```python
from build123d import *

# Parameters (mm, degrees)
SKETCH1_R           = 18.5
BOSS_EXTRUDE1_DEPTH = 21.56
SKETCH2_R           = 6
BOSS_EXTRUDE2_DEPTH = 6
SKETCH3_R           = 3
BOSS_EXTRUDE3_DEPTH = 15
SKETCH4_R           = 1.5
CUT_EXTRUDE1_DEPTH  = 4
SKETCH5_R           = 16.4
BOSS_EXTRUDE4_DEPTH = 34
SKETCH7_R           = 0.75
BOSS_EXTRUDE5_DEPTH = 10
SKETCH8_R           = 0.75
BOSS_EXTRUDE6_DEPTH = 10


with BuildPart() as part:
    # Sketch1 → Boss-Extrude1 (new body)
    with BuildSketch(Plane.XY):
        with Locations((-38.660623091, 1.939719844)):
            Circle(SKETCH1_R)
    extrude(amount=BOSS_EXTRUDE1_DEPTH)

    # Sketch2 → Boss-Extrude2 (add)
    with BuildSketch(Plane.XY.offset(21.56)):
        with Locations((-41.618854638, 10.439653144)):
            Circle(SKETCH2_R)
    extrude(amount=BOSS_EXTRUDE2_DEPTH)

    # Sketch3 → Boss-Extrude3 (add)
    with BuildSketch(Plane.XY.offset(27.56)):
        with Locations((-41.618854638, 10.439653144)):
            Circle(SKETCH3_R)
    extrude(amount=BOSS_EXTRUDE3_DEPTH)

    # Sketch4 → Cut-Extrude1 (cut)
    with BuildSketch(Plane.XY.offset(21.56)):
        with Locations((-35.638553095, 17.248200675)):
            Circle(SKETCH4_R)
    extrude(amount=-CUT_EXTRUDE1_DEPTH, mode=Mode.SUBTRACT)

    # Sketch5 → Boss-Extrude4 (add)
    with BuildSketch(Plane(origin=(0, 0, 0), x_dir=(-1, 0, 0), z_dir=(0, 0, -1))):
        with Locations((38.660623091, 1.939719844)):
            Circle(SKETCH5_R)
    extrude(amount=BOSS_EXTRUDE4_DEPTH)

    # Sketch7 → Boss-Extrude5 (add)
    with BuildSketch(Plane(origin=(0, 0, -34), x_dir=(-1, 0, 0), z_dir=(0, 0, -1))):
        with Locations((47.406680411, 13.79413532)):
            Circle(SKETCH7_R)
    extrude(amount=BOSS_EXTRUDE5_DEPTH)

    # Sketch8 → Boss-Extrude6 (add)
    with BuildSketch(Plane(origin=(0, 0, -34), x_dir=(-1, 0, 0), z_dir=(0, 0, -1))):
        with Locations((48.902224114, 12.582392087)):
            Circle(SKETCH8_R)
    extrude(amount=BOSS_EXTRUDE6_DEPTH)


solid = part.part
```
For this review, take the finished solid that the model builds, in its own axes (mm). A direction names the side the tool comes from. Coordinates: 2 decimals unless noted, no trailing zeros. Write each loop counter-clockwise with the first axis right and the second up, starting at its lowest first coordinate (ties: lowest second). Pieces come first, ordered by that corner, then holes. Notation, with made-up numbers: (-22.5, 48) - (-18.5, 48) arc R18 ccw to (-18.5, 54) - close; hole circle Ø7 at (86.25, 35.25). An arc over 180 degrees is marked (long way). Answer in a Markdown table with one row per item. Add a question column.
Q1. We need section C-C, the plane y = 9. State the section outline as (x, z) points.
Q2. Tool access review of faces 1 (the cylindrical face through (-35.834, 18.735, 19.588)), 2 (the flat face through (-46, -13, 0)), 3 (the cylindrical face through (-30.12, -14.47, 10.63)): name each direction out of +Z, -Z, +X, -X, +Y, -Y from which nothing blocks a thin tool from reaching the whole face with its end or side.
Q3. For P1, Ø10, axis at x = -51, y = 14, coming from the +Z side; P2, Ø6, axis at y = 5.5, z = 8.5, coming from the +X side; P3, Ø2.5, axis at x = -35.64, y = 17.25, coming from the -Z side, all flat-tipped, find the tip position at first contact; note any pin that passes through.
Q4. We need section D-D, the plane z = 13.5. State the section outline as (x, y) points, and give its area (3 significant figures).
Q5. We need section A-A, the plane y = -7. State the section outline as (x, z) points.
Q6. We need section B-B, the plane x = -30. State the section outline as (y, z) points.
Q7. For probe 1 along Z at (x, y) = (-48, -13.5); probe 2 along Z at (x, y) = (-52, 9); probe 3 along X at (y, z) = (14.5, -28.5), list the stretches that pass through material, from the lowest coordinate up.
Q8. Draft analysis for pull direction Y (two halves, no side actions). For faces 4 (the cylindrical face through (-42.27, 7.51, 34.96)), 5 (the flat face through (-36, 17, 17.56)), 6 (the flat face through (-38, 2, -34)), state which applies: +Y half, -Y half, draft (parallel to the pull), parting line (faces both ways), or undercut.
Answer list:
| question | item | result |
|---|---|---|
| 1 | outline | (-55.76, 0) - (-53.46, 0) - (-53.46, -34) - (-23.86, -34) - (-23.86, 0) - (-21.56, 0) - (-21.56, 21.56) - (-35.79, 21.56) - (-35.79, 27.56) - (-38.99, 27.56) - (-38.99, 42.56) - (-44.25, 42.56) - (-44.25, 27.56) - (-47.44, 27.56) - (-47.44, 21.56) - (-55.76, 21.56) - close |
| 2 | face 1 | +Z |
| 2 | face 2 | -Z |
| 2 | face 3 | +Z, -Z |
| 3 | P1 | stops at z = 27.56 |
| 3 | P2 | stops at x = -20.17 |
| 3 | P3 | stops at z = -34 |
| 4 | outline | circle Ø37 at (-38.66, 1.94) |
| 4 | area | 1,080 mm2 |
| 5 | outline | (-54.86, 0) - (-52.41, 0) - (-52.41, -34) - (-24.91, -34) - (-24.91, 0) - (-22.46, 0) - (-22.46, 21.56) - (-54.86, 21.56) - close |
| 6 | outline | (-14.41, 0) - (-11.99, 0) - (-11.99, -34) - (15.87, -34) - (15.87, 0) - (18.29, 0) - (18.29, 21.56) - (-14.41, 21.56) - close |
| 7 | probe 1 | z = 0 to 21.56 |
| 7 | probe 2 | z = -34 to 21.56 |
| 7 | probe 3 | x = -49.21 to -28.12 |
| 8 | face 4 | parting line |
| 8 | face 5 | undercut |
| 8 | face 6 | draft |
